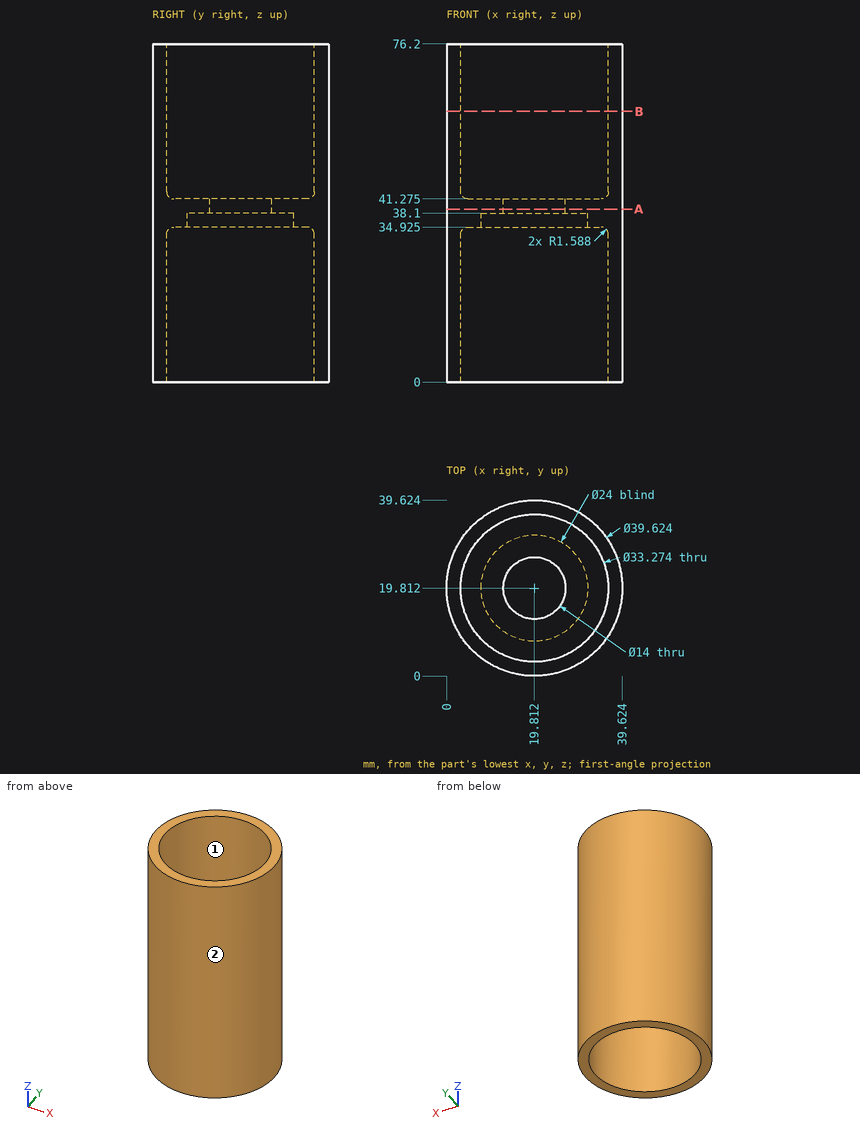
For this review, use the dimensioned drawing (mm, ordinates from the lowest corner) and the shaded views. Give positions to 0.01 mm unless a question says otherwise; leave off trailing zeros. Loops run counter-clockwise (first coordinate to the right, second up) from the corner with the lowest first, then second, coordinate; pieces in that order, holes last.
Item 1: Take a section at A-A, the plane z = 39. State the section outline as (x, y) points (1 decimal), and give its area (3 significant figures).
Item 2: Take a section at B-B, the plane z = 61. State the section outline as (x, y) points (1 decimal).
Item 3: For line 1 along Y through (x, z) = (19.5, 10); line 2 along X through (y, z) = (26, 42) (1 decimal); line 3 along X through (y, z) = (8.5, 47) (1 decimal), list the stretches that pass through material, from the lowest coordinate up.
Item 4: Insertion check: pin 1 (5 mm diameter, centred on x = 13, z = 18, fed in from +Y); pin 2 (10 mm diameter, centred on y = 10, z = 18, fed in from -X); pin 3 (2 mm diameter, centred on y = 35.5, z = 59.5, fed in from +X). Each pin has a flat end and moves straight along its axis. Give the tip position at first contact, or say it passes through.
Item 5: Draft analysis for pull direction Y (two halves, no side actions). For the marked faces 1 and 2, state which applies: +Y half, -Y half, draft (parallel to the pull), parting line (faces both ways), or undercut.
Calculated:
1. outline: circle Ø39.6 at (19.8, 19.8); hole circle Ø14 at (19.8, 19.8)
1. area: 1,080 mm2
2. outline: circle Ø39.6 at (19.8, 19.8); hole circle Ø33.3 at (19.8, 19.8)
3. line 1: y = 0 to 3.18, 36.45 to 39.62
3. line 2: x = 1 to 4.6, 35 to 38.6
3. line 3: x = 3.5 to 7.6, 32 to 36.1
4. pin 1: stops at y = 39.15
4. pin 2: stops at x = 0.59
4. pin 3: stops at x = 33.11
5. face 1: undercut
5. face 2: parting line
